Source: CAD feature listing. Evaluate the final solid. Frame: model axes, mm. Round coordinates to 2 decimals unless told otherwise and drop trailing zeros. Loops run counter-clockwise (first coordinate to the right, second up) from the corner with the lowest first, then second, coordinate; pieces in that order, holes last. Notation, with made-up numbers: (-8, 86.25) - (18, 86.25) arc R24 ccw to (18, 114.25) - close; hole circle Ø5 at (-8.5, 8.25). An arc over 180 degrees is marked (long way). One line per question, with ' | ' between items. Start each with the question number.
1. Pin query (flat end, axial travel): pin 1 (4 mm diameter, centred on x = -70.5, z = -4, fed in from +Y). Return the tip coordinate at first contact, or that it passes through.
2. Cut plane D-D (y = -11). Return loops of the section in (x, z).
3. Ray query, line 1 (Y direction, x = 40, z = -7.25); line 2 (Z direction, x = -71, y = 20); line 3 (Y direction, x = 12, z = -2.5). Return the intervals inside material, ascending.
4. Cut plane A-A (y = 0). Return loops of the section in (x, z).
5. Cut plane B-B (x = -71). Return loops of the section in (y, z), then the cut area to 3 significant figures.
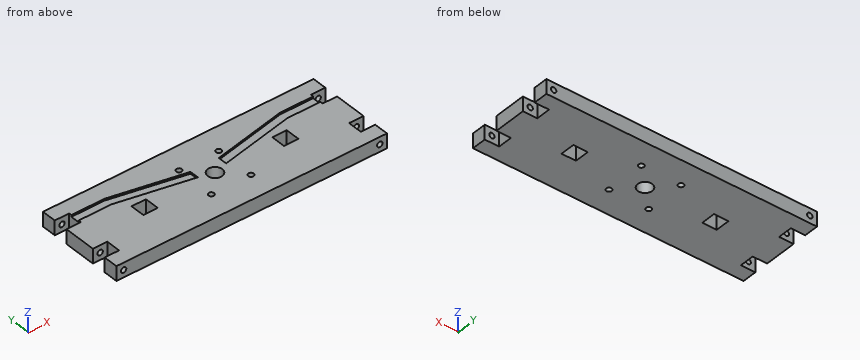
```python
from build123d import *

# Parameters (mm, degrees)
SKETCH1_W                                  = 150
SKETCH1_H                                  = 50
U_ARM_BOTTOM_BOSS_EXTRUDE1_DEPTH           = 8
SKETCH2_W                                  = 8
SKETCH2_H                                  = 8
PUZZLE_SLOT_CUT_EXTRUDE1_DEPTH             = 8
SKETCH3_R                                  = 4
CENTER_SHAFT_HOLE_CUT_EXTRUDE2_DEPTH       = 8
PUZZLE_SLOT_SCREW_HOLES_CUT_EXTRUDE3_REACH = 92.493
SKETCH4_R                                  = 1.5
SIDE_PUZZLE_SLOTS_CUT_EXTRUDE4_DEPTH       = 8
CABLE_CUT_EXTRUDE13_DEPTH                  = 1
SKETCH7_R                                  = 1.5
DISTANS_MOUNTING_HOLES_CUT_EXTRUDE1_DEPTH  = 8


with BuildPart() as part:
    # Sketch1 → U-Arm Bottom Boss-Extrude1 (new body)
    with BuildSketch(Plane.XY):
        Rectangle(SKETCH1_W, SKETCH1_H)
    extrude(amount=-U_ARM_BOTTOM_BOSS_EXTRUDE1_DEPTH)

    # Sketch2 → Puzzle Slot Cut-Extrude1 (cut)
    with BuildSketch(Plane.XY):
        with Locations((71, 13)):
            Rectangle(SKETCH2_W, SKETCH2_H)
        with Locations((71, -13)):
            Rectangle(SKETCH2_W, SKETCH2_H)
        with Locations((-71, -13)):
            Rectangle(SKETCH2_W, SKETCH2_H)
        with Locations((-71, 13)):
            Rectangle(SKETCH2_W, SKETCH2_H)
    extrude(amount=-PUZZLE_SLOT_CUT_EXTRUDE1_DEPTH, mode=Mode.SUBTRACT)

    # Sketch3 → Center Shaft Hole Cut-Extrude2 (cut)
    with BuildSketch(Plane.XY):
        Circle(SKETCH3_R)
    extrude(amount=-CENTER_SHAFT_HOLE_CUT_EXTRUDE2_DEPTH, mode=Mode.SUBTRACT)

    # Puzzle Slot Screw Holes Cut-Extrude3: up to this face of the body (flat: up to its plane)
    puzzle_slot_screw_holes_cut_extrude3_end = Plane(part.part.faces().sort_by_distance((0, 25, -4))[0])
    # Sketch4 → Puzzle Slot Screw Holes Cut-Extrude3 (cut, up to the picked face)
    with BuildSketch(Plane.XZ.offset(25), mode=Mode.PRIVATE) as puzzle_slot_screw_holes_cut_extrude3_sk1:
        with Locations(Location((-71, -4, 0), (0, 0, 90))):
            Circle(SKETCH4_R)
    puzzle_slot_screw_holes_cut_extrude3_tool1 = split(extrude(puzzle_slot_screw_holes_cut_extrude3_sk1.sketch, amount=-PUZZLE_SLOT_SCREW_HOLES_CUT_EXTRUDE3_REACH, mode=Mode.PRIVATE), bisect_by=puzzle_slot_screw_holes_cut_extrude3_end, keep=Keep.BOTH, mode=Mode.PRIVATE)
    # Sketch4 → Puzzle Slot Screw Holes Cut-Extrude3 (cut, up to the picked face)
    with BuildSketch(Plane.XZ.offset(25), mode=Mode.PRIVATE) as puzzle_slot_screw_holes_cut_extrude3_sk2:
        with Locations((71, -4)):
            Circle(SKETCH4_R)
    puzzle_slot_screw_holes_cut_extrude3_tool2 = split(extrude(puzzle_slot_screw_holes_cut_extrude3_sk2.sketch, amount=-PUZZLE_SLOT_SCREW_HOLES_CUT_EXTRUDE3_REACH, mode=Mode.PRIVATE), bisect_by=puzzle_slot_screw_holes_cut_extrude3_end, keep=Keep.BOTH, mode=Mode.PRIVATE)
    add(puzzle_slot_screw_holes_cut_extrude3_tool1.solids().sort_by(Axis((-71, -25, -4), (0, 1, 0)))[0], mode=Mode.SUBTRACT)
    add(puzzle_slot_screw_holes_cut_extrude3_tool2.solids().sort_by(Axis((71, -25, -4), (0, 1, 0)))[0], mode=Mode.SUBTRACT)

    # Sketch5 → Side Puzzle Slots Cut-Extrude4 (cut)
    with BuildSketch(Plane.XY):
        Polygon((-35, 4), (-35, 0), (-35, -4), (-43, -4), (-43, 4), align=None)
        Polygon((43, 4), (43, -4), (35, -4), (35, 0), (35, 4), align=None)
    extrude(amount=-SIDE_PUZZLE_SLOTS_CUT_EXTRUDE4_DEPTH, mode=Mode.SUBTRACT)

    # Sketch6 → Cable Cut-Extrude13 (cut)
    with BuildSketch(Plane.XY):
        Polygon((67, 15.5), (48.657587673, 15.5), (7.841649412, 7.048524191), (7.841649412, 2.048524191), (48.657587673, 10.5), (67, 10.5), align=None)
        Polygon((-7.841649412, 7.048524191), (-7.841649412, 2.048524191), (-48.657587673, 10.5), (-67, 10.5), (-67, 15.5), (-48.657587673, 15.5), align=None)
    extrude(amount=-CABLE_CUT_EXTRUDE13_DEPTH, mode=Mode.SUBTRACT)

    # Sketch7 → Distans Mounting Holes Cut-Extrude1 (cut)
    with BuildSketch(Plane.XY):
        with Locations((11, 11)):
            Circle(SKETCH7_R)
        with Locations((-11, 11)):
            Circle(SKETCH7_R)
        with Locations((-11, -11)):
            Circle(SKETCH7_R)
        with Locations((11, -11)):
            Circle(SKETCH7_R)
    extrude(amount=-DISTANS_MOUNTING_HOLES_CUT_EXTRUDE1_DEPTH, mode=Mode.SUBTRACT)


solid = part.part
```
Answers follow:
1) pin 1: stops at y = 25
2) outline: (-67, -8) - (-12.5, -8) - (-12.5, 0) - (-67, 0) - close; (-9.5, -8) - (9.5, -8) - (9.5, 0) - (-9.5, 0) - close; (12.5, -8) - (67, -8) - (67, 0) - (12.5, 0) - close
3) line 1: y = -25 to -4, 4 to 25 | line 2: z = -8 to -5.5, -2.5 to 0 | line 3: y = -25 to -12.12, -9.88 to 9.88, 12.12 to 25
4) outline: (-75, -8) - (-43, -8) - (-43, 0) - (-75, 0) - close; (-35, -8) - (-4, -8) - (-4, 0) - (-35, 0) - close; (4, -8) - (35, -8) - (35, 0) - (4, 0) - close; (43, -8) - (75, -8) - (75, 0) - (43, 0) - close; hole circle Ø3 at (-71, -4); hole circle Ø3 at (71, -4)
5) outline: (-25, -8) - (-17, -8) - (-17, -5.5) - (-25, -5.5) - close; (-25, -2.5) - (-17, -2.5) - (-17, 0) - (-25, 0) - close; (-9, -8) - (9, -8) - (9, -5.5) - (-9, -5.5) - close; (-9, -2.5) - (9, -2.5) - (9, 0) - (-9, 0) - close; (17, -8) - (25, -8) - (25, -5.5) - (17, -5.5) - close; (17, -2.5) - (25, -2.5) - (25, 0) - (17, 0) - close | area: 170 mm2
